```python
from build123d import *

# Parameters (mm, degrees)
F0_W          = 50
F0_H          = 52
F2_DEPTH      = 30
F1_W          = 43
F1_H          = 43
F3_DEPTH      = 30
F5_W          = 40
F5_H          = 30
F6_DEPTH      = 5.5
F4_W          = 10
F4_H          = 5.5
F7_DEPTH      = 20
F8_R          = 1.5
F9_DEPTH      = 25
F10_R         = 2.75
F11_DEPTH     = 3
F12_T1_DEPTH  = 5.5
F12_T6_DEPTH  = 5.5
F12_T11_DEPTH = 5
F12_T17_DEPTH = 31.2168298797
F12_T22_DEPTH = 30.7168298797
F13_SIZE      = 14.99999
F14_SIZE      = 5
F15_SIZE      = 5


# Not quite as in the source:
# - a fillet or chamfer that OpenCascade refuses, or shapes differently, is made with other operations: its cross-section is extruded or revolved along the edge and cut away or added
# - a fillet or chamfer is up to 0.001 mm smaller than in the source, because OpenCascade refuses the exact size


with BuildPart() as f2:
    # F0 (on Front) → F2 (new body)
    with BuildSketch(Plane.XZ):
        with Locations((0, -1)):
            Rectangle(F0_W, F0_H)
    extrude(amount=F2_DEPTH)

    # F1 (on face) → F3 (cut)
    with BuildSketch(Plane.XZ):
        Rectangle(F1_W, F1_H)
    extrude(amount=F3_DEPTH, mode=Mode.SUBTRACT)

    # F5 (on face) → F6 (join)
    with BuildSketch(Plane.XY.offset(-21.5)):
        with Locations((-15, -40)):
            Rectangle(F5_W, F5_H)
    extrude(amount=-F6_DEPTH)

    # F4 (on face) → F7 (join)
    with BuildSketch(Plane.XZ.offset(30)):
        with Locations((-20, -24.25)):
            Rectangle(F4_W, F4_H)
    extrude(amount=F7_DEPTH)

    # F8 (on face) → F9 (cut)
    with BuildSketch(Plane.XY.offset(-21.5)):
        with Locations((-20, -45)):
            Circle(F8_R)
        with Locations((13.5, -25)):
            Circle(F8_R)
    extrude(amount=-F9_DEPTH, mode=Mode.SUBTRACT)

    # F10 (on face) → F11 (cut)
    with BuildSketch(Plane.XY.offset(-21.5)):
        with Locations((-20, -45)):
            Circle(F10_R)
        with Locations((13.5, -25)):
            Circle(F10_R)
    extrude(amount=-F11_DEPTH, mode=Mode.SUBTRACT)

    # F12: chamfer of 10 on 3 edges, made by hand

    # F12_s2 → F12_t1 (join)
    with BuildSketch(Plane.XY.offset(-27)):
        Polygon((15, -30), (5, -40), (5, -30), align=None)
    extrude(amount=F12_T1_DEPTH)


with BuildPart() as f12_tool4:
    # F12_s5 → F12_t6 (new body)
    with BuildSketch(Plane.XY.offset(-27)):
        Polygon((-25, -15), (-35, -25), (-25, -25), align=None)
    extrude(amount=F12_T6_DEPTH)

    split(bisect_by=Plane.YZ.offset(-35), keep=Keep.TOP)


with BuildPart() as f2_1:
    add(f2.part)

    # F12_t3: union F12_tool4
    add(f12_tool4.part)


with BuildPart() as f12_tool9:
    # F12_s10 → F12_t11 (new body)
    with BuildSketch(Plane.XZ.offset(25)):
        Polygon((-25, -11.5), (-35, -21.5), (-25, -21.5), align=None)
    extrude(amount=F12_T11_DEPTH)

    split(bisect_by=Plane.YZ.offset(-35), keep=Keep.TOP)


with BuildPart() as f2_2:
    add(f2_1.part)

    # F12_t8: union F12_tool9
    add(f12_tool9.part)


with BuildPart() as f12_tool15:
    # F12_s16 → F12_t17 (new body)
    with BuildSketch(Plane.XY.offset(-27)):
        Polygon((-25, -15), (-35, -25), (-25, -25), align=None)
    extrude(amount=F12_T17_DEPTH)

    split(bisect_by=Plane.XY.offset(-21.5), keep=Keep.TOP)

    split(bisect_by=Plane.YZ.offset(-35), keep=Keep.TOP)


with BuildPart() as f12_tool20:
    # F12_s21 → F12_t22 (new body)
    with BuildSketch(Plane.XZ.offset(-0.7168298797)):
        Polygon((-25, -11.5), (-35, -21.5), (-25, -21.5), align=None)
    extrude(amount=F12_T22_DEPTH)

    split(bisect_by=Plane.XZ, keep=Keep.TOP)

    split(bisect_by=Plane.XZ.offset(25), keep=Keep.BOTTOM)

    split(bisect_by=Plane.YZ.offset(-35), keep=Keep.TOP)


with BuildPart() as f12_tool15_1:
    add(f12_tool15.part)

    # F12_t26: intersect F12_tool20
    add(f12_tool20.part, mode=Mode.INTERSECT)


with BuildPart() as f2_3:
    add(f2_2.part)

    # F12_t13: union F12_tool15
    add(f12_tool15_1.part)

    # F13 (size 15 in the source; OpenCascade refuses exactly that, so slightly less here)
    f13_edges = [f2_3.edges().sort_by_distance(p)[0] for p in [
        (5, -55, -24.25),
    ]]
    chamfer(f13_edges, length=F13_SIZE)

    # F14
    f14_edges = [f2_3.edges().sort_by_distance(p)[0] for p in [
        (-35, -55, -24.25),
    ]]
    chamfer(f14_edges, length=F14_SIZE)

    # F15
    f15_edges = [f2_3.edges().sort_by_distance(p)[0] for p in [
        (-35, -25, -24.25),
    ]]
    chamfer(f15_edges, length=F15_SIZE)


solid = f2_3.part
```
Work out the finished part from the listing and answer in its coordinate system (mm). A direction names the side the tool comes from. Round coordinates to 2 decimals unless told otherwise and drop trailing zeros. Loops run counter-clockwise (first coordinate to the right, second up) from the corner with the lowest first, then second, coordinate; pieces in that order, holes last. Notation, with made-up numbers: M 33,81 L 72,81 A32 cw 72,114 Z; hole C -25.5,-4.5 d11. An arc over 180 degrees is marked long. Use CSV: the item, a comma, the result in double quotes.
Q1. Consider L1, parallel to Z at x = 16, y = -5; L2, parallel to X at y = -20.5, z = -11.5; L3, parallel to Y at x = 22.5, z = -4.5. Determine where each line is inside the solid, lowest interval first.
Determined:
L1,"-27 to -21.5, 21.5 to 25"
L2,"-25 to -21.5, 21.5 to 25"
L3,"-30 to 0"
Q2. The mould has two halves that part along Z. Classify faces 6 (the flat face through (0, -15, 25)), 7 (the flat face through (-33.207, -25.672, -23.423)), 8 (the flat face through (-7, -27, -21.5)): pulls with the +Z half, pulls with the -Z half, needs draft (parallel to the pull), parting line crosses it, or undercut.
Determined:
face 6,"pulls with the +Z half"
face 7,"needs draft"
face 8,"undercut"
Q3. Section A-A, the plane y = -8.5 is taken. Determine the outline of the cut face in (x, z), then the cut area to 3 significant figures.
Determined:
outline,"M -25,-27 L 25,-27 L 25,25 L -25,25 Z; hole M -21.5,-21.5 L 21.5,-21.5 L 21.5,21.5 L -21.5,21.5 Z"
area,"751 mm2"
Q4. Section D-D, the plane z = -23 is taken. State how many separate pieces and enclosed holes the cut face has, then the cut area to 3 significant figures.
Determined:
separate pieces,"1"
enclosed holes,"2"
area,"2,470 mm2"
Q5. Each of these flat-tipped pins is pushed along its axis until it touches: pin 1 (6 mm diameter, centred on x = -19, y = -44.5, fed in from +Z); pin 2 (5 mm diameter, centred on x = -20, y = -45, fed in from +Z); pin 3 (9 mm diameter, centred on y = -17.5, z = -3.5, fed in from -X). Where does it stop, or does it pass through?
Determined:
pin 1,"z = -21.5"
pin 2,"z = -24.5"
pin 3,"x = -25"
Q6. Section C-C, the plane x = -20 is taken. Determine the outline of the cut face in (y, z), then the cut area to 4 significant figures.
Determined:
outline,"M -55,-27 L -46.5,-27 L -46.5,-24.5 L -47.75,-24.5 L -47.75,-21.5 L -55,-21.5 Z; M -43.5,-27 L 0,-27 L 0,-21.5 L -42.25,-21.5 L -42.25,-24.5 L -43.5,-24.5 Z; M -30,21.5 L 0,21.5 L 0,25 L -30,25 Z"
area,"383.5 mm2"
Q7. Section B-B, the plane z = 1 is taken. Determine the outline of the cut face in (x, y).
Determined:
outline,"M -25,-30 L -21.5,-30 L -21.5,0 L -25,0 Z; M 21.5,-30 L 25,-30 L 25,0 L 21.5,0 Z"
Q8. A tool of negligible diameter and unlimited length cuts with its end or side. For faces 1 (the cylindrical face through (13.305, -23.513, -25.732)), 2 (the flat face through (-25, -15, 4)), 3 (the cylindrical face through (13.142, -22.273, -22.979)), 4 (the flat face through (0, -15, 21.5)), 5 (the flat face through (25, -15, -1)), from which of +Z, -Z, +X, -X, +Y, -Y can it reach the whole face along a straight path? Write none if from no direction.
Determined:
face 1,"-Z"
face 2,"+Z, -X, +Y"
face 3,"none"
face 4,"+Y, -Y"
face 5,"+Z, -Z, +X, +Y, -Y"
